Input: part model. Units: mm. Frame: model coordinates. Face numbers are marked on the shaded views. A direction names the side the tool comes from. Round coordinates to 2 decimals unless told otherwise and drop trailing zeros. Loops run counter-clockwise (first coordinate to the right, second up) from the corner with the lowest first, then second, coordinate; pieces in that order, holes last. Notation, with made-up numbers: (68.25, 2) -> (96.25, 2) arc R25 cw to (96.25, 21) -> close; hole circle Ø2 at (31.25, -37.5). An arc over 180 degrees is marked (long way). Answer in a Markdown table with one row per item. Add a question column.
Q1. Section C-C, the plane y = 8.5. Output: boundary loops of the cut face in (x, z), and give its area (3 significant figures).
Q2. Section D-D, the plane y = -8. Output: boundary loops of the cut face in (x, z), and give its area (3 significant figures).
Q3. Section B-B, the plane x = 0. Output: boundary loops of the cut face in (y, z), and give its area (3 significant figures).
Q4. Section A-A, the plane z = 5.25. Output: boundary loops of the cut face in (x, y), and give its area (3 significant figures).
Q5. Ray query, L1, parallel to X at y = 10.5, z = 3.5; L2, parallel to Z at x = 5.5, y = -1; L3, parallel to X at y = -6, z = 8.5. Return the intervals inside material, ascending. Write a range as from..to.
Q6. Pin query (flat end, axial travel): pin 1 (8 mm diameter, centred on x = -5, y = 4.5, fed in from +Z); pin 2 (2 mm diameter, centred on y = 6, z = 1, fed in from -X); pin 3 (1.5 mm diameter, centred on x = -12.5, y = 7.5, fed in from -Z); pin 4 (3 mm diameter, centred on y = 5, z = 8.5, fed in from +X). Return the tip coordinate at first contact, or that it passes through.
Q7. Reachability of the marked faces 5, 6 and 7 from +Z, -Z, +X, -X, +Y, -Y: full face, straight path, thin tool, end or side. Return the list, or none.
Q8. Mould query, pull axis X, two halves, no side actions, for the marked faces 1, 2, 3 and 4. Classes: pulls with the +X half, pulls with the -X half, needs draft (parallel to the pull), parting line crosses it, or undercut.
```python
from build123d import *

# Parameters (mm, degrees)
PAD_DEPTH            = 9.5
POCKET_DEPTH         = 1.7
POCKET001_DEPTH      = 100
POCKET001_DEPTH_BACK = 100
POCKET002_DEPTH      = 2.5
POCKET003_DEPTH      = 100
POCKET003_DEPTH_BACK = 100
PAD001_DEPTH         = 31.5


with BuildPart() as part:
    # Sketch → Pad (new body)
    with BuildSketch(Plane.XY):
        with BuildLine():
            ThreePointArc((15.75, 0), (0, 15.75), (-15.75, 0))
            Line((-15.75, 0), (-15.75, -32))
            Line((-15.75, -32), (15.75, -32))
            Line((15.75, 0), (15.75, -32))
        make_face()
    extrude(amount=PAD_DEPTH)

    # Sketch002 (on Face6 of Pad) → Pocket (cut)
    with BuildSketch(Plane.XY.offset(9.5)):
        with BuildLine():
            ThreePointArc((-6.75, 0), (0, -6.75), (6.75, 0))
            Line((6.75, 0), (6.75, 32))
            Line((-6.75, 32), (6.75, 32))
            Line((-6.75, 0), (-6.75, 32))
        make_face()
    extrude(amount=-POCKET_DEPTH, mode=Mode.SUBTRACT)

    # Sketch001 (on Face6 of Pad) → Pocket001 (cut, two sides)
    with BuildSketch(Plane.XY.offset(9.5)) as pocket001_sk:
        with BuildLine():
            ThreePointArc((-5.25, 0), (0, -5.25), (5.25, 0))
            Line((5.25, 0), (5.25, 32))
            Line((-5.25, 32), (5.25, 32))
            Line((-5.25, 0), (-5.25, 32))
        make_face()
    extrude(amount=-POCKET001_DEPTH, mode=Mode.SUBTRACT)
    extrude(pocket001_sk.sketch, amount=POCKET001_DEPTH_BACK, mode=Mode.SUBTRACT)

    # Sketch003 (on Face2 of Pocket001) → Pocket002 (cut)
    with BuildSketch(Plane(origin=(0, 0, 0), x_dir=(1, 0, 0), z_dir=(0, 0, -1))):
        with BuildLine():
            ThreePointArc((10.25, 0), (0, 10.25), (-10.25, 0))
            Line((-10.25, 0), (-10.25, -32))
            Line((-10.25, -32), (10.25, -32))
            Line((10.25, 0), (10.25, -32))
        make_face()
    extrude(amount=-POCKET002_DEPTH, mode=Mode.SUBTRACT)

    # Sketch004 (on Face11 of Pocket002) → Pocket003 (cut, two sides)
    with BuildSketch(Plane(origin=(-15.75, 0, 0), x_dir=(0, -1, 0), z_dir=(-1, 0, 0))) as pocket003_sk:
        Polygon((12, 0), (32, 2.5), (32, 0), align=None)
    extrude(amount=-POCKET003_DEPTH, mode=Mode.SUBTRACT)
    extrude(pocket003_sk.sketch, amount=POCKET003_DEPTH_BACK, mode=Mode.SUBTRACT)

    # Sketch005 (on Face11 of Pocket003) → Pad001 (join)
    with BuildSketch(Plane(origin=(-15.75, 0, 0), x_dir=(0, -1, 0), z_dir=(-1, 0, 0))):
        Polygon((12, 9.5), (32, 12), (32, 9.5), align=None)
    extrude(amount=-PAD001_DEPTH)


solid = part.part
```
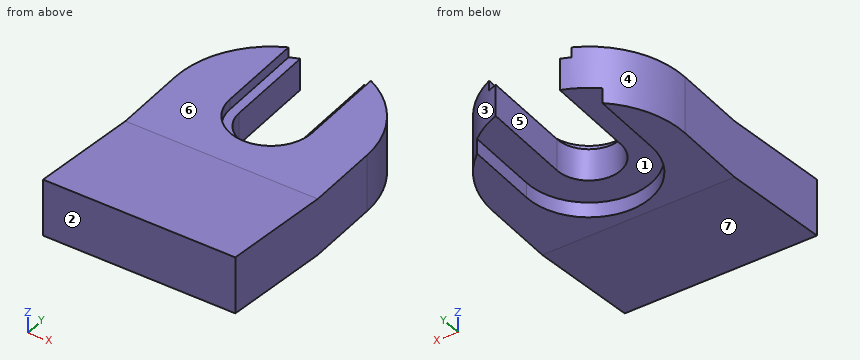
Answer block:
| question | item | result |
|---|---|---|
| 1 | outline | (-13.26, 0) -> (-10.25, 0) -> (-10.25, 2.5) -> (-5.25, 2.5) -> (-5.25, 7.8) -> (-6.75, 7.8) -> (-6.75, 9.5) -> (-13.26, 9.5) -> close; (5.25, 2.5) -> (10.25, 2.5) -> (10.25, 0) -> (13.26, 0) -> (13.26, 9.5) -> (6.75, 9.5) -> (6.75, 7.8) -> (5.25, 7.8) -> close |
| 1 | area | 122 mm^2 |
| 2 | outline | (-15.75, 0) -> (-6.41, 0) -> (-6.41, 2.5) -> (6.41, 2.5) -> (6.41, 0) -> (15.75, 0) -> (15.75, 9.5) -> (-15.75, 9.5) -> close |
| 2 | area | 267 mm^2 |
| 3 | outline | (-32, 2.5) -> (-12, 0) -> (-10.25, 0) -> (-10.25, 2.5) -> (-5.25, 2.5) -> (-5.25, 7.8) -> (-6.75, 7.8) -> (-6.75, 9.5) -> (-12, 9.5) -> (-32, 12) -> close |
| 3 | area | 239 mm^2 |
| 4 | outline | (-15.75, -32) -> (15.75, -32) -> (15.75, 0) arc R15.75 ccw to (5.25, 14.85) -> (5.25, 0) arc R5.25 cw to (-5.25, 0) -> (-5.25, 14.85) arc R15.75 ccw to (-15.75, 0) -> close |
| 4 | area | 1,190 mm^2 |
| 5 | L1 | -11.74..-5.25, 5.25..11.74 |
| 5 | L2 | 2.5..7.8 |
| 5 | L3 | -15.75..-3.09, 3.09..15.75 |
| 6 | pin 1 | z = 9.5 |
| 6 | pin 2 | x = -14.94 |
| 6 | pin 3 | z = 0 |
| 6 | pin 4 | x = 15.36 |
| 7 | face 5 | +Z, -Z, +Y |
| 7 | face 6 | +Z, +X, -X, +Y |
| 7 | face 7 | -Z, +X, -X, -Y |
| 8 | face 1 | undercut |
| 8 | face 2 | needs draft |
| 8 | face 3 | pulls with the +X half |
| 8 | face 4 | pulls with the -X half |
